Check sheet for the drawn part. Datum: minimum x, y, z corner. Units: mm. Round coordinates to 2 decimals unless told otherwise and drop trailing zeros. Order: outer loops, then holes, each group sorted by start corner. A loop starts at its lowest first (then second) coordinate and runs counter-clockwise, first axis right, second up. Notation, with made-up numbers: M 20.25,53 L 66.25,53 A19 cw 66.25,89 Z; hole C -20,81.25 d4. An arc over 180 degrees is marked long. Use one line per item in the form item = value. Start each with the question number.
Item 1: Cross-section at C-C on z = 50. Enter the section's corners in (x, y) (1 decimal).
Item 2: Cross-section at A-A on x = 750.5. Enter the section's corners in (y, z) (1 decimal).
Item 3: Go/stop test with flat-tipped pins: pin 1 Ø8 at (x, z) = (553.5, 82.5) entering from -Y; pin 2 Ø1.5 at (x, z) = (657.5, 146) entering from +Y; pin 3 Ø4 at (x, z) = (631.5, 68) entering from +Y. Record where each tip stops, or that it passes through.
Item 4: Cross-section at B-B on y = 103. Enter the section's corners in (x, z).
Item 5: Cross-section at D-D on y = 154.5. Enter the section's corners in (x, z), then the cut area to 3 significant figures.
Item 6: Thickness scan on probe 1 along Y at (x, z) = (370, 24.5) (1 decimal); probe 2 along Z at (x, y) = (386, 116) (1 decimal); probe 3 along Y at (x, z) = (124, 60) (1 decimal). Record the ranges inside material, lowest first. Write a range as [from, to].
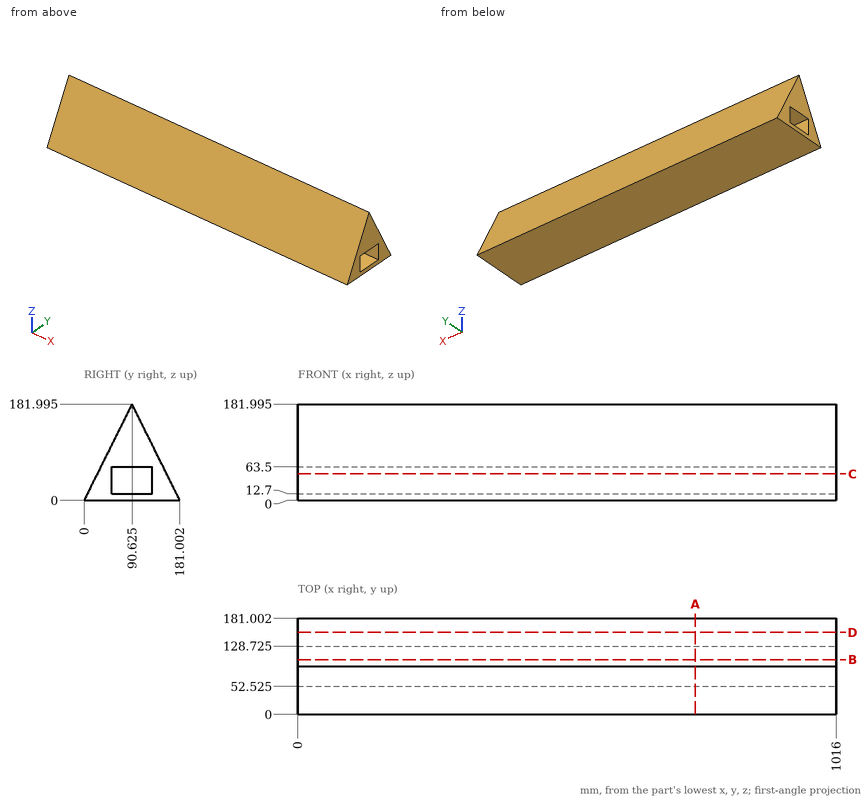
Output values:
q1.outline = M 0,24.9 L 1016,24.9 L 1016,52.5 L 0,52.5 Z; M 0,128.7 L 1016,128.7 L 1016,156.2 L 0,156.2 Z
q2.outline = M 0,0 L 181,0 L 90.6,182 Z; hole M 52.5,12.7 L 128.7,12.7 L 128.7,63.5 L 52.5,63.5 Z
q3.pin_1 = 39.09
q3.pin_2 = 108.87
q3.pin_3 = 148.23
q4.outline = M 0,0 L 1016,0 L 1016,12.7 L 0,12.7 Z; M 0,63.5 L 1016,63.5 L 1016,157.08 L 0,157.08 Z
q5.outline = M 0,0 L 1016,0 L 1016,53.37 L 0,53.37 Z
q5.area = 54,200 mm2
q6.probe_1 = [12.2, 52.5], [128.7, 168.8]
q6.probe_2 = [0, 12.7], [63.5, 130.9]
q6.probe_3 = [29.9, 52.5], [128.7, 151.2]
